from build123d import *

# Parameters (mm, degrees)
BOSS_EXTRUDE2_DEPTH = 10
CIRPATTERN1_COUNT   = 10
SKETCH1_5_R         = 13
BOSS_EXTRUDE3_DEPTH = 10
SKETCH2_R           = 2.5
CUT_EXTRUDE1_DEPTH  = 11


with BuildPart() as part:
    # Sketch1 → Boss-Extrude2 (new body)
    with BuildSketch(Plane(origin=(0, 0, 0), x_dir=(1, 0, 0), z_dir=(0, 1, 0))):
        with BuildLine():
            ThreePointArc((2.628362747, 18.377642448), (0.987757529, 16.436868415), (0, 14.095389312))
            Line((0, 14.095389312), (0, 13))
            ThreePointArc((0, 13), (2.702851981, 12.71591881), (5.28757636, 11.876090949))
            Line((5.28757636, 11.876090949), (5.733111332, 12.876778879))
            ThreePointArc((5.733111332, 12.876778879), (5.783115278, 15.41758366), (5.073731749, 17.857863221))
            Line((5.073731749, 17.857863221), (2.628362747, 18.377642448))
        make_face()
    extrude(amount=BOSS_EXTRUDE2_DEPTH)


with BuildPart() as cirpattern1_1:
    # CirPattern1: pattern copy
    add(part.part.rotate(Axis((0, 0, 0), (0, 1, 0)), 1 * 360 / CIRPATTERN1_COUNT))


with BuildPart() as cirpattern1_2:
    # CirPattern1: pattern copy
    add(part.part.rotate(Axis((0, 0, 0), (0, 1, 0)), 2 * 360 / CIRPATTERN1_COUNT))


with BuildPart() as cirpattern1_3:
    # CirPattern1: pattern copy
    add(part.part.rotate(Axis((0, 0, 0), (0, 1, 0)), 3 * 360 / CIRPATTERN1_COUNT))


with BuildPart() as cirpattern1_4:
    # CirPattern1: pattern copy
    add(part.part.rotate(Axis((0, 0, 0), (0, 1, 0)), 4 * 360 / CIRPATTERN1_COUNT))


with BuildPart() as cirpattern1_5:
    # CirPattern1: pattern copy
    add(part.part.rotate(Axis((0, 0, 0), (0, 1, 0)), 5 * 360 / CIRPATTERN1_COUNT))


with BuildPart() as cirpattern1_6:
    # CirPattern1: pattern copy
    add(part.part.rotate(Axis((0, 0, 0), (0, 1, 0)), 6 * 360 / CIRPATTERN1_COUNT))


with BuildPart() as cirpattern1_7:
    # CirPattern1: pattern copy
    add(part.part.rotate(Axis((0, 0, 0), (0, 1, 0)), 7 * 360 / CIRPATTERN1_COUNT))


with BuildPart() as cirpattern1_8:
    # CirPattern1: pattern copy
    add(part.part.rotate(Axis((0, 0, 0), (0, 1, 0)), 8 * 360 / CIRPATTERN1_COUNT))


with BuildPart() as cirpattern1_9:
    # CirPattern1: pattern copy
    add(part.part.rotate(Axis((0, 0, 0), (0, 1, 0)), 9 * 360 / CIRPATTERN1_COUNT))


with BuildPart() as part_1:
    add(part.part)

    add(cirpattern1_1.part)  # Boss-Extrude3 merges CirPattern1_1

    add(cirpattern1_2.part)  # Boss-Extrude3 merges CirPattern1_2

    add(cirpattern1_3.part)  # Boss-Extrude3 merges CirPattern1_3

    add(cirpattern1_4.part)  # Boss-Extrude3 merges CirPattern1_4

    add(cirpattern1_5.part)  # Boss-Extrude3 merges CirPattern1_5

    add(cirpattern1_6.part)  # Boss-Extrude3 merges CirPattern1_6

    add(cirpattern1_7.part)  # Boss-Extrude3 merges CirPattern1_7

    add(cirpattern1_8.part)  # Boss-Extrude3 merges CirPattern1_8

    add(cirpattern1_9.part)  # Boss-Extrude3 merges CirPattern1_9
    # Sketch1_5 → Boss-Extrude3 (add)
    with BuildSketch(Plane(origin=(0, 0, 0), x_dir=(1, 0, 0), z_dir=(0, 1, 0))):
        Circle(SKETCH1_5_R)
    extrude(amount=BOSS_EXTRUDE3_DEPTH)

    # Sketch2 → Cut-Extrude1 (cut, through all)
    with BuildSketch(Plane.XZ):
        Circle(SKETCH2_R)
    extrude(amount=-CUT_EXTRUDE1_DEPTH, mode=Mode.SUBTRACT)


solid = part_1.part
Design review of the part built by this model. Coordinates are the model's own, in mm. A direction names the side the tool comes from. Give positions to 0.01 mm unless a question says otherwise; leave off trailing zeros. Loops run counter-clockwise (first coordinate to the right, second up) from the corner with the lowest first, then second, coordinate; pieces in that order, holes last. Notation, with made-up numbers: (64.25, 4) - (94.25, 4) arc R30 ccw to (94.25, 32) - close; hole circle Ø10 at (29, -4.5). An arc over 180 degrees is marked (long way). Write item = value, one per line.
1) To check wall thickness, follow line 1 (Z direction, x = 15, y = 5); line 2 (X direction, y = 7.5, z = 9); line 3 (Z direction, x = 13.5, y = 1). State the ranges of each line that lie inside material, in increasing order.
Result sheet:
line_1 = -4.31 to 1.27, 5.66 to 10.38
line_2 = -13.7 to 9.38, 10 to 16.19
line_3 = -12.69 to -8.66, -4.36 to 1.42, 4.42 to 10.36
2) Tool access review of faces 4 (the face through (0, 4.9, -13.6)), 5 (the face through (-7.97, 4.93, 10.97)), 6 (the face through (11.726, 4.93, -6.77)), 7 (the face through (-12.89, 4.93, 4.19)): name each direction out of +Z, -Z, +X, -X, +Y, -Y from which nothing blocks a thin tool from reaching the whole face with its end or side.
Result sheet:
face_4 = -Z, +Y, -Y
face_5 = +Z, +Y, -Y
face_6 = +X, +Y, -Y
face_7 = +Y, -Y
3) Clearance check with flat-ended pins moving along their axes: pin 1 Ø2 at (x, y) = (-10.5, 1.5) entering from -Z; pin 2 Ø0.9 at (y, z) = (5.5, -13.5) entering from -X; pin 3 Ø1 at (x, y) = (7.5, 1.5) entering from +Z. State where each tip first meets the part, or that it passes through.
Result sheet:
pin_1 = -9.89
pin_2 = -8.87
pin_3 = 17.16
4) Take a section at A-A on z = 0. State the section outline as (x, y) points.
Result sheet:
outline = (-17.7, 0) - (-2.5, 0) - (-2.5, 10) - (-17.7, 10) - close; (2.5, 0) - (17.7, 0) - (17.7, 10) - (2.5, 10) - close
5) Draft analysis for pull direction X (two halves, no side actions). For faces 1 (the face through (13.78, 4.93, -12.38)), 2 (the face through (-16.42, 4.93, -0.75)), 3 (the face through (-12.841, 4.93, -10.258)), state which applies: +X half, -X half, draft (parallel to the pull), parting line (faces both ways), or undercut.
Result sheet:
face_1 = +X half
face_2 = -X half
face_3 = undercut
6) Take a section at B-B on z = 7.5. State the section outline as (x, y) points, and give its area (3 significant figures).
Result sheet:
outline = (-12.64, 0) - (16.34, 0) - (16.34, 10) - (-12.64, 10) - close
area = 290 mm2
